Verification items for the finished model (mm, model axes). A direction names the side the tool comes from. Coordinates: 2 decimals unless noted, no trailing zeros. Write each loop counter-clockwise with the first axis right and the second up, starting at its lowest first coordinate (ties: lowest second). Pieces come first, ordered by that corner, then holes. Notation, with made-up numbers: (10.5, 73.25) -> (18.5, 73.25) arc R12 cw to (18.5, 84.25) -> close; hole circle Ø6 at (23, -26.75). An arc over 180 degrees is marked (long way). Answer in a Markdown table with one row per item.
```python
from build123d import *

# Parameters (mm, degrees)
AUFSATZ_LINEAR_AUSTRAGEN1_DEPTH = 67.8
SKIZZE3_W                       = 33
SKIZZE3_H                       = 7.6
SKIZZE3_H_2                     = 16.35
SCHNITT_LINEAR_AUSTRAGEN1_DEPTH = 9.1
SKIZZE4_W                       = 2.75
SKIZZE4_H                       = 30.2
AUFSATZ_LINEAR_AUSTRAGEN2_DEPTH = 66.1
VERRUNDUNG1_R                   = 2.75
VERRUNDUNG3_R                   = 1
SCHNITT_LINEAR_AUSTRAGEN2_DEPTH = 35


with BuildPart() as part:
    # Skizze1 → Aufsatz-Linear austragen1 (new body)
    with BuildSketch(Plane(origin=(0, 0, 0), x_dir=(0, 0, -1), z_dir=(1, 0, 0))):
        Polygon((-67.1, 29.991702941), (3.049987553, 29.791286266), (3.049987553, 32.695849754), (0, 32.704563488), (0, 40.304563488), (-9, 40.304563488), (-9, 32.725724599), (-70, 32.9), (-70, -3.1), (-9.1, -2.926010297), (-9.1, -18.44), (0, -18.44), (0, 0), (-67.1, -0.191702941), align=None)
    extrude(amount=-AUFSATZ_LINEAR_AUSTRAGEN1_DEPTH)

    # Skizze3 → Schnitt-Linear austragen1 (cut)
    with BuildSketch(Plane.XY):
        with Locations((-33.95, 36.504563488)):
            Rectangle(SKIZZE3_W, SKIZZE3_H)
        with Locations((-33.95, -10.265)):
            Rectangle(SKIZZE3_W, SKIZZE3_H_2)
    extrude(amount=SCHNITT_LINEAR_AUSTRAGEN1_DEPTH, mode=Mode.SUBTRACT)

    # Skizze4 → Aufsatz-Linear austragen2 (add)
    with BuildSketch(Plane.XY.offset(1)):
        with Locations((-33.625, 15.1)):
            Rectangle(SKIZZE4_W, SKIZZE4_H)
    extrude(amount=AUFSATZ_LINEAR_AUSTRAGEN2_DEPTH)

    # Verrundung1
    verrundung1_edges = [part.edges().sort_by_distance(p)[0] for p in [
        (-59.125, -18.44, 9.1),
        (-59.125, -2.926010297, 9.1),
        (-59.125, 40.304563488, 9),
        (-8.725, 40.304563488, 9),
        (-17.45, 40.304563488, 4.5),
        (-50.45, 40.304563488, 4.5),
        (-8.725, -2.926010297, 9.1),
        (-8.725, -18.44, 9.1),
        (-17.45, -18.44, 4.55),
        (-50.45, -18.44, 4.55),
    ]]
    fillet(verrundung1_edges, radius=VERRUNDUNG1_R)

    # Verrundung3
    verrundung3_edges = [part.edges().sort_by_distance(p)[0] for p in [
        (-33.9, -3.1, 70),
        (-33.9, 32.9, 70),
    ]]
    fillet(verrundung3_edges, radius=VERRUNDUNG3_R)

    # Skizze6 → Schnitt-Linear austragen2 (cut)
    with BuildSketch(Plane(origin=(0, 0, 0), x_dir=(0, 0, -1), z_dir=(1, 0, 0))):
        Polygon((-67.1, 29.991702941), (-34, 29.897137109), (-34, -0.097137109), (-67.1, -0.191702941), align=None)
    extrude(amount=-SCHNITT_LINEAR_AUSTRAGEN2_DEPTH, mode=Mode.SUBTRACT)


solid = part.part
```
1. Section check A-A, the plane y = -9.5. Record the boundary of the cut face in (x, z).
Geometry says:
| item | result |
|---|---|
| outline | (-67.8, 0) -> (-50.45, 0) -> (-50.45, 9.1) -> (-67.8, 9.1) -> close; (-17.45, 0) -> (0, 0) -> (0, 9.1) -> (-17.45, 9.1) -> close |
2. Thickness scan on line 1 (Y direction, x = -17.5, z = 2.5); line 2 (Z direction, x = -33.5, y = 21); line 3 (Z direction, x = -49, y = 24). Record the ranges inside material, lowest first. Write a range as from..to.
Geometry says:
| item | result |
|---|---|
| line 1 | -2.09..-0.01, 29.81..32.7 |
| line 2 | 1..34, 67.1..70 |
| line 3 | 67.1..70 |
3. Section check D-D, the plane y = 34.5. Record the boundary of the cut face in (x, z).
Geometry says:
| item | result |
|---|---|
| outline | (-67.8, 0) -> (-50.45, 0) -> (-50.45, 9) -> (-67.8, 9) -> close; (-17.45, 0) -> (0, 0) -> (0, 9) -> (-17.45, 9) -> close |
4. Depth check by flat-ended pin: P1, Ø8, axis at x = -24.5, y = -7.5, coming from the -Z side; P2, Ø4, axis at x = -53.5, z = 20.5, coming from the -Y side; P3, Ø0.7, axis at x = -35.5, y = -2.5, coming from the -Z side; P4, Ø15, axis at y = 10.5, z = 11, coming from the -X side. Enter the tip coordinate at first touch or a pass-through.
Geometry says:
| item | result |
|---|---|
| P1 | through |
| P2 | y = -2.96 |
| P3 | z = 9.1 |
| P4 | x = -35 |
5. Tool access check on faces 1 (the flat face through (-9, -11, 9.1)), 2 (the flat face through (-34, 15, 34)), 3 (the flat face through (-34, 15, 1)), 4 (the flat face through (-50.45, -9, 5)). Record the directions out of +Z, -Z, +X, -X, +Y, -Y that give a thin tool (end or side, any length) a straight path to the whole face; none if there is none.
Geometry says:
| item | result |
|---|---|
| face 1 | +Z, +X, -X, -Y |
| face 2 | +X, -X |
| face 3 | -Z, +X, -X |
| face 4 | -Z, -Y |
6. Section check C-C, the plane z = 15.5. Record the boundary of the cut face in (x, y).
Geometry says:
| item | result |
|---|---|
| outline | (-67.8, -2.94) -> (0, -2.94) -> (0, -0.04) -> (-67.8, -0.04) -> close; (-67.8, 29.84) -> (-35, 29.84) -> (-35, 0) -> (-32.25, 0) -> (-32.25, 29.84) -> (0, 29.84) -> (0, 32.74) -> (-67.8, 32.74) -> close |
7. Mould release check, pull along X, two halves, no side actions. Record for faces 5 (the cylindrical face through (-16.62, -17.66, 4.61)), 6 (the cylindrical face through (-59.246, -3.715, 9.93)), 7 (the flat face through (0, -2, 34)): released by +X, released by -X, zero draft, split by the parting line, or undercut.
Geometry says:
| item | result |
|---|---|
| face 5 | undercut |
| face 6 | zero draft |
| face 7 | released by +X |
